Input: part model. Units: mm. Frame: model coordinates. Coordinates: 2 decimals unless noted, no trailing zeros. Order: outer loops, then holes, each group sorted by start corner. A loop starts at its lowest first (then second) coordinate and runs counter-clockwise, first axis right, second up. Notation, with made-up numbers: (-27, -24.75) - (18, -24.75) arc R15 cw to (18, -20.75) - close; hole circle Ø6 at (10.25, 7). An arc over 180 degrees is marked (long way). Answer as CSV lines item,"result". Start each with the question number.
Item 1: Material intervals for line 1 along X through (y, z) = (1.15, 50.5); line 2 along Z through (x, y) = (-42, 1.6); line 3 along X through (y, z) = (0.5, -66.5), sorted ascending.
Item 2: Section C-C (x = 47). Output: boundary loops of the cut face in (y, z).
Item 3: Section B-B (y = 1.5). State how many separate pieces and enclosed holes the cut face has, and give its area (3 significant figures).
Item 4: First-contact query: pin 1 (1.5 mm diameter, centred on y = 2, z = 57, fed in from +X); pin 2 (0.9 mm diameter, centred on x = 62.5, y = 1.5, fed in from +Z); pin 3 (0.9 mm diameter, centred on y = 2, z = -72, fed in from +X). Flat tips, straight axial feed; report the tip coordinate or a pass-through.
Item 5: Section A-A (z = 51). Output: boundary loops of the cut face in (x, y).
Autodesk Inventor part; units mm, degrees
ref_plane "YZ Plane" through (0, 0, 0) normal (1, 0, 0) x (0, 1, 0)
ref_plane "XZ Plane" through (0, 0, 0) normal (0, 1, 0) x (-1, 0, 0)
ref_plane "XY Plane" through (0, 0, 0) normal (0, 0, 1) x (1, 0, 0)
sketch "Sketch2" plane through (0, 0, 0) normal (0, 1, 0) x (-1, 0, 0)
  line L0 (-89, 99) -> (89, 99)
  line L1 (89, 99) -> (89, -99)
  line L2 (89, -99) -> (-89, -99)
  line L3 (-89, -99) -> (-89, 99)
  line L4 (-89, 99) -> (89, -99) construction
  line L5 (89, 99) -> (-89, -99) construction
  line L6 (-89, 99) -> (89, 99)
  line L7 (89, 99) -> (89, -85)
  line L8 (89, -85) -> (-89, -85)
  line L9 (-89, -85) -> (-89, 99)
  line L10 (-4.5, 99) -> (-89, 99)
  line L11 (-89, 99) -> (-89, 42)
  line L12 (-89, 42) -> (-4.5, 42)
  line L13 (-4.5, 42) -> (-4.5, 99)
  line L14 (4.5, 99) -> (89, 99)
  line L15 (89, 99) -> (89, 42)
  line L16 (89, 42) -> (4.5, 42)
  line L17 (4.5, 42) -> (4.5, 99)
  line L18 (22.5, 77.5) -> (22.5, 66.5)
  line L19 (16.5, 66.5) -> (16.5, 77.5)
  line L20 (-22.5, 66.5) -> (-22.5, 77.5)
  line L21 (-16.5, 77.5) -> (-16.5, 66.5)
  line L22 (-23.5, 99) -> (-16.5, 99)
  line L23 (-16.5, 99) -> (-16.5, 42)
  line L24 (-16.5, 42) -> (-23.5, 42)
  line L25 (-23.5, 42) -> (-23.5, 99)
  line L26 (16.5, 99) -> (23.5, 99)
  line L27 (23.5, 99) -> (23.5, 42)
  line L28 (23.5, 42) -> (16.5, 42)
  line L29 (16.5, 42) -> (16.5, 99)
  line L30 (-89, 99) -> (89, 99)
  line L31 (89, 99) -> (89, 97)
  line L32 (89, 97) -> (-89, 97)
  line L33 (-89, 97) -> (-89, 99)
  line L34 (89, -85) -> (74, -85)
  line L35 (74, -85) -> (74, -64)
  line L36 (74, -64) -> (89, -64)
  line L37 (89, -64) -> (89, -85)
  line L38 (-89, -85) -> (-74, -85)
  line L39 (-74, -85) -> (-74, -64)
  line L40 (-74, -64) -> (-89, -64)
  line L41 (-89, -64) -> (-89, -85)
  line L42 (16.5, 97) -> (-16.5, 97)
  line L43 (-16.5, 97) -> (-16.5, 93)
  line L44 (-16.5, 93) -> (16.5, 93)
  line L45 (16.5, 93) -> (16.5, 97)
  line L46 (-84.4, -75) -> (-84.4, -71.5)
  line L47 (-84.4, -71.5) -> (-87, -71.5)
  line L48 (-87, -71.5) -> (-87, -75)
  line L49 (-87, -75) -> (-84.4, -75)
  line L50 (-79.6, -75) -> (-77, -75)
  line L51 (-77, -75) -> (-77, -71.5)
  line L52 (-77, -71.5) -> (-79.6, -71.5)
  line L53 (-79.6, -71.5) -> (-79.6, -75)
  line L54 (-75, -78) -> (-89, -78)
  line L55 (-89, -78) -> (-89, -63)
  line L56 (-89, -63) -> (-75, -63)
  line L57 (-75, -63) -> (-75, -78)
  circle A0 centre (-80.45, -67.25) radius 1.25
  point P0 (0, 0)
  point P1 (4.5, 99)
  point P2 (-4.5, 99)
  point P3 (-89, 42)
  point P4 (89, 42)
  point P5 (4.5, 97)
  point P6 (-4.5, 97)
  point P7 (-16.5, 97)
  point P8 (-23.5, 97)
  point P9 (23.5, 97)
  point P10 (16.5, 98)
  point P11 (-4.5, 93)
  point P12 (4.5, 93)
  point P13 (16.5, 93)
  dimension "d8" = 178
  dimension "d9" = 198
  dimension "d10" = 14
  dimension "d11" = 84.5
  dimension "d13" = 84.5
  dimension "d17" = 9
  dimension "d18" = 2
  dimension "d19" = 15
  dimension "d20" = 21
  dimension "d21" = 15
  dimension "d22" = 21
  dimension "d75" = 55
  dimension "d76" = 55
  dimension "d77" = 7
  dimension "d78" = 7
  dimension "d79" = 4
extrude "Extrusion2" add sketch "Sketch2" along normal blind 3 contours L32 L23 L21 L12 L25 | L12 L13 L44 L17 L16 L1 L36 L35 L8 L39 L40 L57 L56 L3 | L32 L13 L44 L23 | L56 L57 L40 L3 | L32 L17 L44 L13 | L32 L29 L44 L17 | L32 L27 L16 L29 L19
fillet "Fillet5" radius 3 12 edges at (-16.5, 1.5, 42) (-4.5, 1.5, 42) (-23.5, 1.5, 42) (16.5, 1.5, 42) (-16.5, 1.5, 93) (-4.5, 1.5, 93) (4.5, 1.5, 93) (16.5, 1.5, 93) (4.5, 1.5, 42) (23.5, 1.5, 42) (74, 1.5, -64) (-74, 1.5, -64)
equation "\"d11\" = d13"
properties part number "base" material "Aluminum 6061"
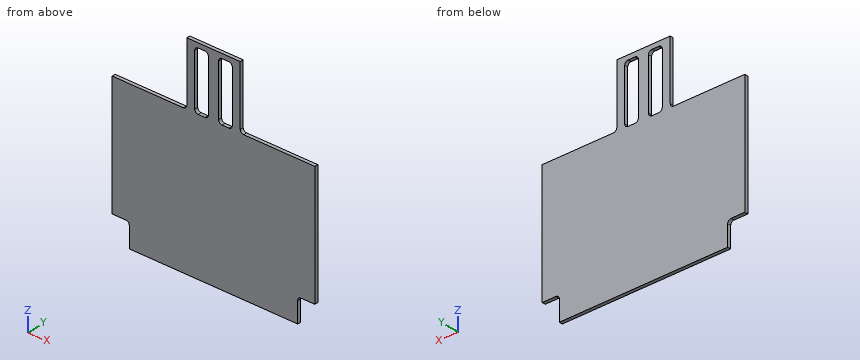
Determined:
1,line 1,"x = -23.5 to -16.5, -4.5 to 4.5, 16.5 to 23.5"
1,line 2,"z = -85 to 42"
1,line 3,"x = -74.04 to 74.04"
2,outline,"(0, -85) - (3, -85) - (3, 42) - (0, 42) - close"
3,separate pieces,"1"
3,enclosed holes,"2"
3,area,"23,400 mm^2"
4,pin 1,"stops at x = 23.5"
4,pin 2,"stops at z = 42"
4,pin 3,"stops at x = 74"
5,outline,"(-23.5, 0) - (-16.5, 0) - (-16.5, 3) - (-23.5, 3) - close; (-4.5, 0) - (4.5, 0) - (4.5, 3) - (-4.5, 3) - close; (16.5, 0) - (23.5, 0) - (23.5, 3) - (16.5, 3) - close"
